Part model, mm, in its own coordinate system. A direction names the side the tool comes from. Round coordinates to 2 decimals unless told otherwise and drop trailing zeros. Write each loop counter-clockwise with the first axis right and the second up, starting at its lowest first coordinate (ties: lowest second). Pieces come first, ordered by that corner, then holes. Notation, with made-up numbers: (69, 23) -> (98, 23) arc R30 ccw to (98, 57) -> close; hole circle Ø2 at (6, -9.5). An arc over 180 degrees is marked (long way). Use CSV: the item, a comma, the result in double quotes. Start each with the question number.
(1) Saw through at D-D (x = -41). Give the cut face in (y, z).
(2) Probe line 1 (Y direction, x = 58, z = -21.5); line 2 (Z direction, x = 9.5, y = -15.25); line 3 (Z direction, x = 13, y = -24.5). List the from-to ranges inside material, lowest first. Write a range as [from, to].
(3) Two-plate mould, pull along Z, no slides. Class faces 1 (the cylindrical face through (49.23, -12.88, -2.33)), 2 (the flat face through (-1, -5, -28.558)), 3 (the flat face through (18.8, -25.4, -18.4)): released by +Z, released by -Z, zero draft, split by the parting line, or undercut.
(4) Saw through at C-C (y = -13.5). Give the cut face in (x, z), plus the area to 3 significant figures.
(5) Drop flat-ended pins along their axis: pin 1 (5 mm diameter, centred on y = -17.5, z = 35.5, fed in from -X); pin 2 (3 mm diameter, centred on y = -19.5, z = -19.5, fed in from +X). Give the stop position or say it passes through.
(6) Which spindle directions (+Z, -Z, +X, -X, +Y, -Y) get a long thin tool onto all of the face, cutting with end or side? Do faces 4 (the flat face through (-8, -15, -12.473)), 5 (the flat face through (-10, -16, 23.132)), 6 (the cylindrical face through (56.33, -17.93, 14.51)). Say none if no direction does.
(7) Saw through at A-A (z = -2). Give the cut face in (x, y), plus the area to 3 significant figures.
(8) Saw through at B-B (x = 40.5). Give the cut face in (y, z).
```python
from build123d import *

# Parameters (mm, degrees)
F1_R     = 31.75
F1_R_2   = 24.309091266
F2_DEPTH = 25.4
F0_W     = 142.668440938
F0_H     = 77.8410565108
F3_DEPTH = 10.668
F5_DEPTH = 14.224
F7_DEPTH = 37.846
F8_DEPTH = 25.4


with BuildPart() as f2:
    # F1 (on Front) → F2 (new body)
    with BuildSketch(Plane.XZ):
        with Locations((26.0463114828, 4.9752164632)):
            Circle(F1_R)
        with Locations((26.0463114828, 4.9752164632)):
            Circle(F1_R_2, mode=Mode.SUBTRACT)
    extrude(amount=F2_DEPTH)

    # F0 (on Front) → F3 (join)
    with BuildSketch(Plane.XZ):
        with Locations((0.12049824, 10.3627415374)):
            Rectangle(F0_W, F0_H)
    extrude(amount=F3_DEPTH)

    # F4 (on face) → F5 (join)
    with BuildSketch(Plane.XZ.offset(10.668)):
        with BuildLine():
            ThreePointArc((-0.4795487258, -12.4730281532), (-5.7008090732, 5.4028102), (0, 23.1315420315))
            Line((0, 23.1315420315), (-27.0918570459, 23.1315420315))
            Line((-27.0918570459, 23.1315420315), (-27.0918570459, -12.4730281532))
            Line((-27.0918570459, -12.4730281532), (-0.4795487258, -12.4730281532))
        make_face()
    extrude(amount=F5_DEPTH)

    # F6 (on face) → F7 (cut)
    with BuildSketch(Plane(origin=(0, 0, -12.4730281532), x_dir=(1, 0, 0), z_dir=(0, 0, -1))):
        Polygon((-27.0918570459, 10.668), (-0.4795487258, 24.892), (-27.0918570459, 24.892), align=None)
    extrude(amount=-F7_DEPTH, mode=Mode.SUBTRACT)

    # F8 (cut): a face of the model
    f8_faces = [f2.faces().sort_by_distance(p)[0] for p in [
        (26.0463114828, -10.668, 4.9752164632),
    ]]
    extrude(f8_faces, amount=-F8_DEPTH, mode=Mode.SUBTRACT)


solid = f2.part
```
Answers:
1,outline,"(-10.67, -28.56) -> (0, -28.56) -> (0, 49.28) -> (-10.67, 49.28) -> close"
2,line 1,"y = [-10.67, 0]"
2,line 2,"z = [-22.12, -12.83], [22.78, 32.07]"
2,line 3,"z = [-23.97, -15.54], [25.49, 33.92]"
3,face 1,"undercut"
3,face 2,"released by -Z"
3,face 3,"zero draft"
4,outline,"(-21.79, -12.47) -> (-0.48, -12.47) arc R31.75 ccw (long way) to (0, 23.13) -> (-21.79, 23.13) -> close; hole circle Ø48.62 at (26.05, 4.98)"
4,area,"1,950 mm²"
5,pin 1,"stops at x = 11.12"
5,pin 2,"stops at x = 47.96"
6,face 4,"-Z, -X, -Y"
6,face 5,"+Z, -X, -Y"
6,face 6,"-Y"
7,outline,"(-71.21, -10.67) -> (-27.09, -10.67) -> (-0.48, -24.89) -> (-4.93, -24.89) -> (-4.93, -25.4) -> (2.76, -25.4) -> (2.76, 0) -> (-71.21, 0) -> close; (49.33, -25.4) -> (57.02, -25.4) -> (57.02, -10.67) -> (71.45, -10.67) -> (71.45, 0) -> (49.33, 0) -> close"
7,area,"1,380 mm²"
8,outline,"(-25.4, -23.29) -> (-10.67, -23.29) -> (-10.67, -28.56) -> (0, -28.56) -> (0, -14.57) -> (-25.4, -14.57) -> close; (-25.4, 24.52) -> (0, 24.52) -> (0, 49.28) -> (-10.67, 49.28) -> (-10.67, 33.24) -> (-25.4, 33.24) -> close"
